Print and shaded views of the part. All mm, measured from the part's lowest x, y and z. Give positions to 0.01 mm unless a question says otherwise; leave off trailing zeros. Order: outer loops, then holes, each group sorted by start corner. A loop starts at its lowest first (then second) coordinate and runs counter-clockwise, first axis right, second up. Notation, with made-up numbers: (42, 63) - (72, 63) arc R23 cw to (72, 102) - close; hole circle Ø7 at (-3.5, 66). An arc over 180 degrees is marked (long way). Answer in a Markdown table with one row per item.
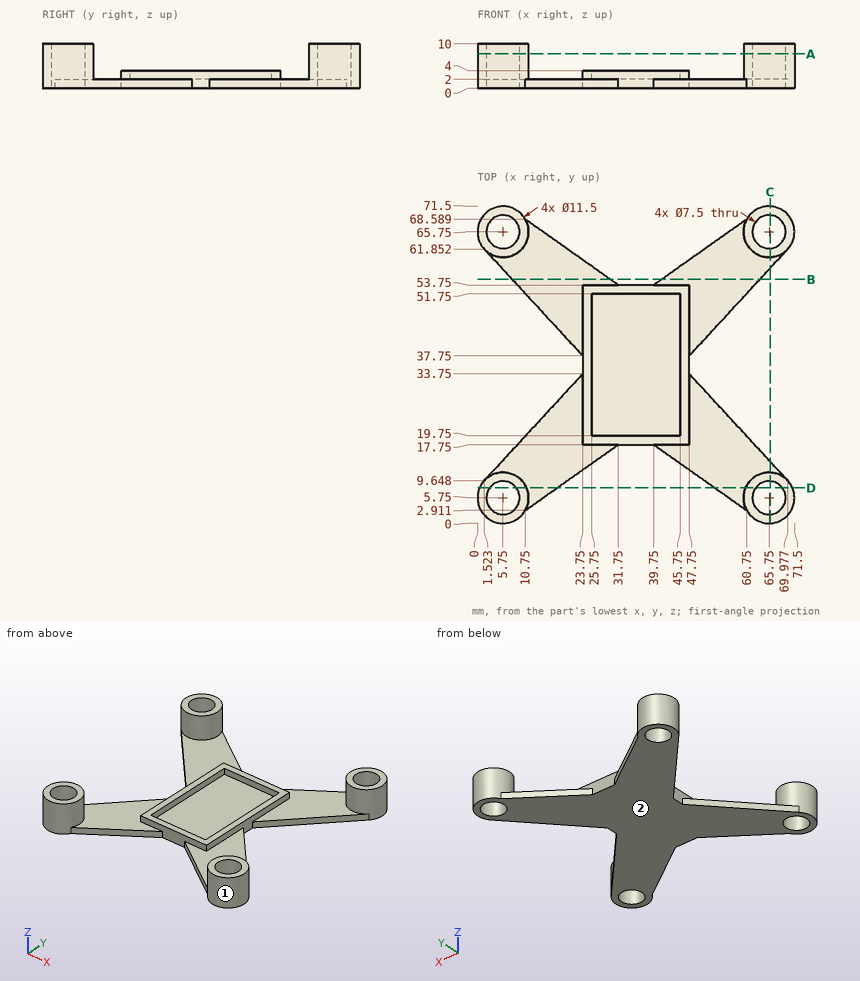
1. Probe line 1 (Y direction, x = 5.75, z = 5); line 2 (Y direction, x = 67, z = 4) (1 decimal); line 3 (Z direction, x = 54, y = 8). List the from-to ranges inside material, lowest first.
Check result:
| item | result |
|---|---|
| line 1 | y = 0 to 2, 9.5 to 11.5, 60 to 62, 69.5 to 71.5 |
| line 2 | y = 0.1 to 2.2, 9.3 to 11.4, 60.1 to 62.2, 69.3 to 71.4 |
| line 3 | z = 0 to 2 |
2. Cut at B-B on y = 55. Write the cut outline in (x, z).
Check result:
| item | result |
|---|---|
| outline | (7.84, 0) - (29.98, 0) - (29.98, 2) - (7.84, 2) - close; (41.52, 0) - (63.66, 0) - (63.66, 2) - (41.52, 2) - close |
3. Cut at A-A on z = 7.75. Write the cut outline in (x, y), and give its area (3 significant figures).
Check result:
| item | result |
|---|---|
| outline | circle Ø11.5 at (5.75, 5.75); circle Ø11.5 at (5.75, 65.75); circle Ø11.5 at (65.75, 5.75); circle Ø11.5 at (65.75, 65.75); hole circle Ø7.5 at (5.75, 5.75); hole circle Ø7.5 at (5.75, 65.75); hole circle Ø7.5 at (65.75, 5.75); hole circle Ø7.5 at (65.75, 65.75) |
| area | 239 mm² |
4. Two-plate mould, pull along X, no slides. Class the marked faces 1 and 2: +X half, -X half, draft (parallel to the pull), parting line (faces both ways), or undercut.
Check result:
| item | result |
|---|---|
| face 1 | undercut |
| face 2 | draft |
5. Cut at D-D on y = 8. Write the cut outline in (x, z).
Check result:
| item | result |
|---|---|
| outline | (0.46, 0) - (2.75, 0) - (2.75, 10) - (0.46, 10) - close; (8.75, 0) - (17.95, 0) - (17.95, 2) - (11.04, 2) - (11.04, 10) - (8.75, 10) - close; (53.55, 0) - (62.75, 0) - (62.75, 10) - (60.46, 10) - (60.46, 2) - (53.55, 2) - close; (68.75, 0) - (71.04, 0) - (71.04, 10) - (68.75, 10) - close |
6. Drop flat-ended pins along their axis: P1, Ø6, axis at y = 31.5, z = 2.5, coming from the -X side; P2, Ø24, axis at x = 59.5, y = 56.5, coming from the +Z side; P3, Ø1, axis at x = 33, z = 3, coming from the -Y side; P4, Ø0.6, axis at y = 28.5, z = 3, coming from the +X side. Give the stop position or say it passes through.
Check result:
| item | result |
|---|---|
| P1 | stops at x = 18.95 |
| P2 | stops at z = 10 |
| P3 | stops at y = 17.75 |
| P4 | stops at x = 47.75 |
7. Cut at C-C on x = 66. Write the cut outline in (y, z) (1 decimal).
Check result:
| item | result |
|---|---|
| outline | (0, 0) - (2, 0) - (2, 10) - (0, 10) - close; (9.5, 0) - (14, 0) - (14, 2) - (11.5, 2) - (11.5, 10) - (9.5, 10) - close; (57.5, 0) - (62, 0) - (62, 10) - (60, 10) - (60, 2) - (57.5, 2) - close; (69.5, 0) - (71.5, 0) - (71.5, 10) - (69.5, 10) - close |
